```python
from build123d import *

# Parameters (mm, degrees)
BOSS_EXTRUDE1_DEPTH = 57.15
FILLET1_R           = 6.35
FILLET2_R           = 6.35


with BuildPart() as part:
    # Sketch2 → Boss-Extrude1 (new body)
    with BuildSketch(Plane.XY):
        Polygon((0, 0), (0, 38.1), (-3.175, 50.396722124), (-38.1, 87.286888497), (-39.169814825, 86.274063497), (-4.506325115, 49.660122124), (-1.4732, 37.912879066), (-1.4732, 0), align=None)
    extrude(amount=-BOSS_EXTRUDE1_DEPTH)

    # Fillet1
    fillet1_edges = [part.edges().sort_by_distance(p)[0] for p in [
        (-3.175, 50.396722124, -28.575),
        (0, 38.1, -28.575),
    ]]
    fillet(fillet1_edges, radius=FILLET1_R)

    # Fillet2
    fillet2_edges = [part.edges().sort_by_distance(p)[0] for p in [
        (-1.4732, 37.912879066, -28.575),
        (-4.506325115, 49.660122124, -28.575),
    ]]
    fillet(fillet2_edges, radius=FILLET2_R)


solid = part.part
```
Input: part model. Units: mm. Frame: model coordinates. A direction names the side the tool comes from. Coordinates: 2 decimals unless noted, no trailing zeros. Loops run counter-clockwise (first coordinate to the right, second up) from the corner with the lowest first, then second, coordinate; pieces in that order, holes last.
Q1. Section B-B, the plane y = 12. Return the cut outline in (x, z).
Results are:
outline: (-1.47, -57.15) - (0, -57.15) - (0, 0) - (-1.47, 0) - close
Q2. Line query: line 1 along X through (y, z) = (27.5, -51); line 2 along Y through (x, z) = (-30.5, -54); line 3 along Y through (x, z) = (-15, -13). Output: solid intervals per line, ascending.
Results are:
line 1: x = -1.47 to 0
line 2: y = 77.12 to 79.26
line 3: y = 60.74 to 62.89
Q3. Section C-C, the plane x = -12. Return the cut outline in (y, z), and give its area (3 significant figures).
Results are:
outline: (57.58, -57.15) - (59.72, -57.15) - (59.72, 0) - (57.58, 0) - close
area: 122 mm2
Q4. Set-up query: faces 1 (the flat face through (-1.473, 19, -28)), 2 (the flat face through (0, 18, -28)). Return all of +Z, -Z, +X, -X, +Y, -Y with unobstructed straight access to the full face (end or side cutting, diameter ignored); none if empty.
Results are:
face 1: +Z, -Z, -X, -Y
face 2: +Z, -Z, +X, +Y, -Y
Q5. Section A-A, the plane z = -21. Return the cut outline in (x, y), and give its area (3 significant figures).
Results are:
outline: (-39.17, 86.27) - (-5.63, 50.85) arc R6.35 cw to (-4.1, 48.07) - (-1.67, 38.69) arc R6.35 cw to (-1.47, 37.11) - (-1.47, 0) - (0, 0) - (0, 37.29) arc R6.35 ccw to (-0.2, 38.88) - (-2.77, 48.81) arc R6.35 ccw to (-4.3, 51.59) - (-38.1, 87.29) - close
area: 149 mm2
Q6. Contact query for flat-ended pins moving along their axis: pin 1 (1.5 mm diameter, centred on y = 17, z = -29, fed in from -X); pin 2 (4 mm diameter, centred on y = 57, z = -7, fed in from -X); pin 3 (5 mm diameter, centred on x = -6, z = -18.5, fed in from +Y); pin 4 (10 mm diameter, centred on x = -4.5, y = 62.5, fed in from -Z). Output: stop coordinate, or through.
Results are:
pin 1: stops at x = -1.47
pin 2: stops at x = -13.35
pin 3: stops at y = 56.02
pin 4: passes through
